Read the model definition and answer for the solid it produces. Units are mm, in the model's axes. Face numbers are marked on the shaded views. Coordinates: 2 decimals unless noted, no trailing zeros. Loops run counter-clockwise (first coordinate to the right, second up) from the corner with the lowest first, then second, coordinate; pieces in that order, holes last. Notation, with made-up numbers: (15.25, -21) - (61.25, -21) arc R14 ccw to (61.25, 3) - close; hole circle Ø7 at (50, 73). An arc over 180 degrees is marked (long way). Use one line per item in the form item = value.
from build123d import *

# Parameters (mm, degrees)
SKETCH2_W           = 28.513595166
SKETCH2_H           = 20.580060423
BOSS_EXTRUDE1_DEPTH = 46.5
SKETCH3_W           = 28.513595166
SKETCH3_H           = 20.580060423
BOSS_EXTRUDE2_DEPTH = 3


with BuildPart() as part:
    # Sketch2 → Boss-Extrude1 (new body)
    with BuildSketch(Plane.XY):
        with Locations((-1.649546828, 5.419939578)):
            Rectangle(SKETCH2_W, SKETCH2_H)
        with BuildLine():
            Line((-12.649546828, 14.531722054), (9.350453172, 14.531722054))
            ThreePointArc((9.350453172, 14.531722054), (10.764666735, 13.945935617), (11.350453172, 12.531722054))
            Line((11.350453172, 12.531722054), (11.350453172, -0.568277946))
            ThreePointArc((11.350453172, -0.568277946), (10.764666735, -1.982491508), (9.350453172, -2.568277946))
            Line((9.350453172, -2.568277946), (-12.649546828, -2.568277946))
            ThreePointArc((-12.649546828, -2.568277946), (-14.06376039, -1.982491508), (-14.649546828, -0.568277946))
            Line((-14.649546828, -0.568277946), (-14.649546828, 12.531722054))
            ThreePointArc((-14.649546828, 12.531722054), (-14.06376039, 13.945935617), (-12.649546828, 14.531722054))
        make_face(mode=Mode.SUBTRACT)
    extrude(amount=BOSS_EXTRUDE1_DEPTH)

    # Sketch3 → Boss-Extrude2 (add)
    with BuildSketch(Plane.XY.offset(46.5)):
        with Locations((-1.649546828, 5.419939578)):
            Rectangle(SKETCH3_W, SKETCH3_H)
    extrude(amount=BOSS_EXTRUDE2_DEPTH)


solid = part.part
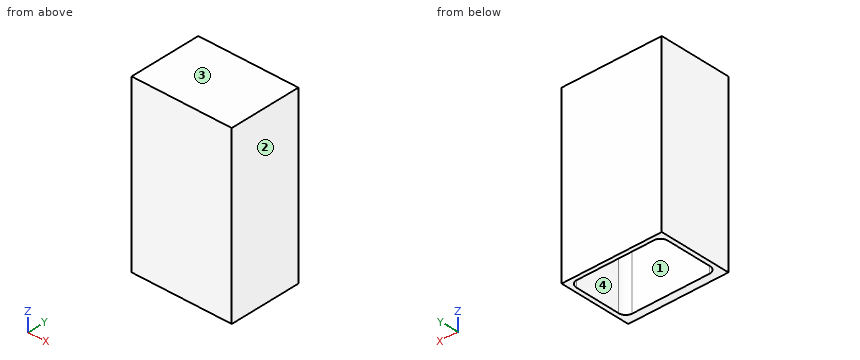
Item 1: Find the intervals of material crossed by L1, parallel to Y at x = 4.25, z = 12; L2, parallel to X at y = 5, z = 30.5; L3, parallel to Z at x = -10.75, y = 2.25, in increasing order.
Results below:
L1 = -4.87 to -2.57, 14.53 to 15.71
L2 = -15.91 to -14.65, 11.35 to 12.61
L3 = 46.5 to 49.5
Item 2: For a pull along X with two mould halves and no side action, classify the marked faces 1, 2, 3 and 4 as +X half, -X half, draft (parallel to the pull), parting line (faces both ways), or undercut.
Results below:
face_1 = undercut
face_2 = +X half
face_3 = draft
face_4 = undercut
Item 3: The part is cut by section C-C on x = -5.25. Give the vertices of the cut face in (y, z), plus the area to 3 significant figures.
Results below:
outline = (-4.87, 0) - (-2.57, 0) - (-2.57, 46.5) - (14.53, 46.5) - (14.53, 0) - (15.71, 0) - (15.71, 49.5) - (-4.87, 49.5) - close
area = 224 mm²
Item 4: This flat-tipped pin is pushed along its axis until it touches: P1, Ø5, axis at x = -0.5, y = 3.5, coming from the -Z side. Where does it stop, or does it pass through?
Results below:
P1 = 46.5
Item 5: The part is cut by section A-A on z = 25.5. Give the vertices of the cut face in (x, y), plus the area to 3 significant figures.
Results below:
outline = (-15.91, -4.87) - (12.61, -4.87) - (12.61, 15.71) - (-15.91, 15.71) - close; hole (-14.65, -0.57) arc R2 ccw to (-12.65, -2.57) - (9.35, -2.57) arc R2 ccw to (11.35, -0.57) - (11.35, 12.53) arc R2 ccw to (9.35, 14.53) - (-12.65, 14.53) arc R2 ccw to (-14.65, 12.53) - close
area = 146 mm²
Item 6: The part is cut by section B-B on y = 10. Give the vertices of the cut face in (x, z), plus the area to 3 significant figures.
Results below:
outline = (-15.91, 0) - (-14.65, 0) - (-14.65, 46.5) - (11.35, 46.5) - (11.35, 0) - (12.61, 0) - (12.61, 49.5) - (-15.91, 49.5) - close
area = 202 mm²
